```python
from build123d import *

# Parameters (mm, degrees)
F1_DEPTH = 62.5
F2_W     = 20
F2_H     = 15
F3_DEPTH = 15.001
F4_DEPTH = 40
F5_R     = 5
F6_DEPTH = 15


with BuildPart() as f1:
    # F0 (on Front) → F1 (new body, symmetric)
    with BuildSketch(Plane.XZ):
        Polygon((-60, -15), (-75, -15), (-75, -90), (-60, -90), (-60, -52.5), align=None)
        with BuildLine():
            Line((-37.5, 0), (-75, 0))
            Line((-75, 0), (-75, -15))
            Line((-75, -15), (-60, -15))
            Line((-60, -15), (-34.3693177122, -15))
            ThreePointArc((-34.3693177122, -15), (-36.7089867349, -7.6616116383), (-37.5, 0))
        make_face()
    extrude(amount=F1_DEPTH, both=True)

    # F2 (on face) → F3 (cut, through all)
    with BuildSketch(Plane.YZ.offset(-60)):
        with Locations((32.4, -82.5)):
            Rectangle(F2_W, F2_H)
        with BuildLine():
            Line((22.4, -75), (42.4, -75))
            ThreePointArc((42.4, -75), (32.4, -65), (22.4, -75))
        make_face()
        with Locations((-32.4, -82.5)):
            Rectangle(F2_W, F2_H)
        with BuildLine():
            Line((-42.4, -75), (-22.4, -75))
            ThreePointArc((-22.4, -75), (-32.4, -65), (-42.4, -75))
        make_face()
    extrude(amount=-F3_DEPTH, mode=Mode.SUBTRACT)

    # F0 (on Front) → F4 (join, symmetric)
    with BuildSketch(Plane.XZ):
        with BuildLine():
            Line((-34.3693177122, -15), (-60, -15))
            Line((-60, -15), (-60, -52.5))
            Line((-60, -52.5), (-10, -36.142080737))
            ThreePointArc((-10, -36.142080737), (-24.5744986324, -28.3256776965), (-34.3693177122, -15))
        make_face()
        with BuildLine():
            Line((-20, -15), (-34.3693177122, -15))
            ThreePointArc((-34.3693177122, -15), (-24.5744986324, -28.3256776965), (-10, -36.142080737))
            ThreePointArc((-10, -36.142080737), (-5.0458880468, -37.1589694935), (0, -37.5))
            Line((0, -37.5), (0, -25))
            ThreePointArc((0, -25), (-11.1803398875, -22.360679775), (-20, -15))
        make_face()
        with BuildLine():
            ThreePointArc((0, -37.5), (-5.0458880468, -37.1589694935), (-10, -36.142080737))
            Line((-10, -36.142080737), (-10, -66.142080737))
            Line((-10, -66.142080737), (0, -66.142080737))
            Line((0, -66.142080737), (0, -37.5))
        make_face()
        with BuildLine():
            Line((-25, 0), (-37.5, 0))
            ThreePointArc((-37.5, 0), (-36.7089867349, -7.6616116383), (-34.3693177122, -15))
            Line((-34.3693177122, -15), (-20, -15))
            ThreePointArc((-20, -15), (-23.7170824513, -7.9056941504), (-25, 0))
        make_face()
    extrude(amount=F4_DEPTH, both=True)

    # F5 (on face) → F6 (cut)
    with BuildSketch(Plane.YZ):
        with Locations((-20, -45.5710403685)):
            Circle(F5_R)
        with Locations((20, -45.5710403685)):
            Circle(F5_R)
    extrude(amount=-F6_DEPTH, mode=Mode.SUBTRACT)


solid = f1.part
```
CAD build for the part. Positions are in the model's coordinates, mm. A direction names the side the tool comes from. Round coordinates to 2 decimals unless told otherwise and drop trailing zeros. Loops run counter-clockwise (first coordinate to the right, second up) from the corner with the lowest first, then second, coordinate; pieces in that order, holes last. Notation, with made-up numbers: M -33,-38.75 L -18,-38.75 A26 ccw -18,-4.75 Z; hole C -21,50.25 d9. An arc over 180 degrees is marked long. Return JSON: item names as keys, results as strings. Group by question number.
(1) Drop flat-ended pins along their axis: P1, Ø5, axis at x = -50, y = 22, coming from the -Z side; P2, Ø10, axis at x = -21, y = -15.5, coming from the -Z side; P3, Ø7, axis at x = -51.5, y = 52.5, coming from the -Z side; P4, Ø16, axis at y = 20, z = -45.57, coming from the +X side. Give the stop position or say it passes through.
(2) Wall check: probe 1 along X at (y, z) = (8.5, -57); probe 2 along X at (y, z) = (51, -16); probe 3 along Y at (x, z) = (-12.5, -25.5). Give the ranges that are in metal, low to high. Write a range as [from, to].
(3) Saw through at D-D, the plane z = -82. List the corners of the cut face in (x, y), and give its area (4 significant figures).
(4) Saw through at B-B, the plane y = -20. List the corners of the cut face in (x, z), and give its area (3 significant figures).
(5) Saw through at A-A, the plane z = -69. List the corners of the cut face in (x, y), and give its area (4 significant figures).
(6) Saw through at C-C, the plane x = -68. List the corners of the cut face in (y, z).
(7) Mould opens along Z. For faces 1 (the cylindrical face through (-4.93, -20.651, -40.614)), 2 (the cylindrical face through (-36.687, 51.092, -7.767)), 3 (the flat face through (-10, -1, -51)) say: +Z half, -Z half, draft (parallel to the pull), parting line (faces both ways), or undercut.
(8) Tool access for faces 4 (the flat face through (-5, -1, -66.142)), 5 (the cylindrical face through (-4.93, 19.349, -40.614)), 6 (the flat face through (-35.35, -0.56, -44.436)), 7 (the flat face through (-47, -51, -15)), 8 (the flat face through (-67, -22.4, -83)): list every direction of +Z, -Z, +X, -X, +Y, -Y with a clear straight run to the whole face (end or side of a thin tool).
Answer list:
{
 "1": {"P1": "z = -50.05", "P2": "z = -41.38", "P3": "z = -15", "P4": "x = 0"},
 "2": {"probe 1": "[-75, -60], [-10, 0]", "probe 2": "[-75, -60]", "probe 3": "[-40, 40]"},
 "3": {"outline": "M -75,-62.5 L -60,-62.5 L -60,-42.4 L -75,-42.4 Z; M -75,-22.4 L -60,-22.4 L -60,22.4 L -75,22.4 Z; M -75,42.4 L -60,42.4 L -60,62.5 L -75,62.5 Z", "area": "1,275 mm2"},
 "4": {"outline": "M -75,-90 L -60,-90 L -60,-52.5 L -10,-36.14 L -10,-40.57 L 0,-40.57 L 0,-25 A25 cw -25,0 L -75,0 Z; M -10,-66.14 L 0,-66.14 L 0,-50.57 L -10,-50.57 Z", "area": "3,640 mm2"},
 "5": {"outline": "M -75,-62.5 L -60,-62.5 L -60,-40.4 L -75,-40.4 Z; M -75,-24.4 L -60,-24.4 L -60,24.4 L -75,24.4 Z; M -75,40.4 L -60,40.4 L -60,62.5 L -75,62.5 Z", "area": "1,395 mm2"},
 "6": {"outline": "M -62.5,-90 L -42.4,-90 L -42.4,-75 A10 cw -22.4,-75 L -22.4,-90 L 22.4,-90 L 22.4,-75 A10 cw 42.4,-75 L 42.4,-90 L 62.5,-90 L 62.5,0 L -62.5,0 Z"},
 "7": {"face 1": "undercut", "face 2": "+Z half", "face 3": "draft"},
 "8": {"face 4": "-Z, +X, +Y, -Y", "face 5": "+X", "face 6": "-Z, +Y, -Y", "face 7": "-Z, +X, -Y", "face 8": "-Z, +X, -X"}
}
